```python
from build123d import *

# Parameters (mm, degrees)
F1_DEPTH = 7.62
F2_DEPTH = 1.27
F4_W     = 50.8
F4_H     = 19.067067
F6_W     = 59.465482
F6_H     = 29.439323
F9_DEPTH = 1.27


with BuildPart() as f1:
    # F0 (on Top) → F1 (new body)
    with BuildSketch(Plane.XY):
        Polygon((12.7, 12.7), (-12.7, 12.7), (-12.7, -38.1), (-12.7, -76.2), (12.7, -76.2), (12.7, -38.1), align=None)
        Polygon((12.7, -76.2), (-12.7, -76.2), (0, -127), align=None)
    extrude(amount=F1_DEPTH)

    # F0 (on Top) → F2 (join)
    with BuildSketch(Plane.XY):
        with BuildLine():
            ThreePointArc((139.7, 0), (77.911288, 23.462884), (12.7, 12.7))
            Line((12.7, 12.7), (12.7, -38.1))
            ThreePointArc((12.7, -38.1), (72.718847, -7.994233), (139.7, -12.7))
            Line((139.7, -12.7), (139.7, 0))
        make_face()
        with BuildLine():
            Line((-12.7, -38.1), (-12.7, 12.7))
            ThreePointArc((-12.7, 12.7), (-77.911288, 23.462884), (-139.7, 0))
            Line((-139.7, 0), (-139.7, -12.7))
            ThreePointArc((-139.7, -12.7), (-72.718847, -7.994233), (-12.7, -38.1))
        make_face()
    extrude(amount=F2_DEPTH)

    # F4 (on offset) → F7 section 0
    with BuildSketch(Plane.XZ.offset(76.2)):
        with Locations((0, 17.153533)):
            Rectangle(F4_W, F4_H)
    # F6 (on offset) → F7 section 1
    with BuildSketch(Plane.XZ.offset(127)):
        with Locations((0.102181, 14.719661)):
            Rectangle(F6_W, F6_H)
    loft(mode=Mode.SUBTRACT)

    # F0 (on Top) + F8 (on face) → F9 (join)
    with BuildSketch(Plane.XY):
        Polygon((12.7, -76.2), (-12.7, -76.2), (0, -127), align=None)
    with BuildSketch(Plane.XY):
        Polygon((0, -127), (-12.7, -76.2), (-52.008614, -151.024356), (-52.008614, -167.176113), align=None)
        Polygon((52.008614, -151.024356), (12.7, -76.2), (0, -127), (52.008614, -167.176113), align=None)
    extrude(amount=F9_DEPTH)


solid = f1.part
```
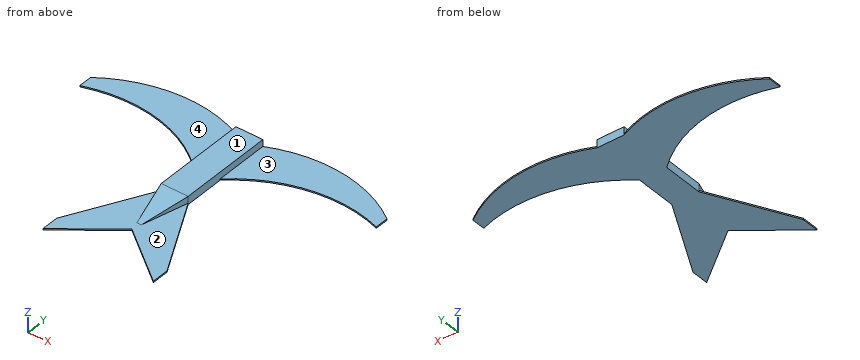
Geometry: final body of the model. Coordinates: model frame, mm. Face numbers are marked on the shaded views. A direction names the side the tool comes from. Coordinates: 2 decimals unless noted, no trailing zeros. Loops run counter-clockwise (first coordinate to the right, second up) from the corner with the lowest first, then second, coordinate; pieces in that order, holes last. Notation, with made-up numbers: (47, 60.25) -> (71, 60.25) arc R18 cw to (71, 86.25) -> close; hole circle Ø8 at (67.5, 48). An arc over 180 degrees is marked (long way). Use a Markdown table: item, result. Add a question column.
(1) Access query for the marked faces 1, 2, 3 and 4. Directions: +Z, -Z, +X, -X, +Y, -Y. A direction counts if a zero-diameter tool reaches every point of the face in a straight line with its end or side. Return the directions, or none.
(2) Section query A-A, the plane x = 16.5. Return loops of the section in (y, z).
(3) Section query D-D, the plane y = -73. Return loops of the section in (x, z), plus the area to 3 significant figures.
(4) Section query C-C, the plane x = 70. Return loops of the section in (y, z).
(5) Section query B-B, the plane y = 4.5. Return loops of the section in (x, z), plus the area to 3 significant figures.
(6) Pin query (flat end, axial travel): pin 1 Ø0.6 at (y, z) = (-162, 0.5) entering from -X; pin 2 Ø4 at (x, z) = (-0.5, 4) entering from +Y; pin 3 Ø1 at (y, z) = (-74, 6) entering from -X; pin 4 Ø3 at (x, z) = (-51, 3.5) entering from -Y. Return the tip coordinate at first contact, or that it passes through.
(7) Line query: line 1 along Z through (x, y) = (-94, 8); line 2 along Y through (x, z) = (-34, 1); line 3 along X through (y, z) = (10.5, 4.5). Output: solid intervals per line, ascending.
Answer:
| question | item | result |
|---|---|---|
| 1 | face 1 | +Z, +X, -X, +Y, -Y |
| 1 | face 2 | +Z, -Y |
| 1 | face 3 | +Z, +X, +Y, -Y |
| 1 | face 4 | +Z, -X, +Y, -Y |
| 2 | outline | (-139.75, 0) -> (-83.43, 0) -> (-83.43, 1.27) -> (-139.75, 1.27) -> close; (-34.82, 0) -> (14.35, 0) -> (14.35, 1.27) -> (-34.82, 1.27) -> close |
| 3 | outline | (-12.7, 0) -> (12.7, 0) -> (12.7, 7.62) -> (-12.7, 7.62) -> close |
| 3 | area | 194 mm^2 |
| 4 | outline | (-8.57, 0) -> (24.01, 0) -> (24.01, 1.27) -> (-8.57, 1.27) -> close |
| 5 | outline | (-133.04, 0) -> (133.04, 0) -> (133.04, 1.27) -> (12.7, 1.27) -> (12.7, 7.62) -> (-12.7, 7.62) -> (-12.7, 1.27) -> (-133.04, 1.27) -> close |
| 5 | area | 499 mm^2 |
| 6 | pin 1 | stops at x = -52.01 |
| 6 | pin 2 | stops at y = 12.7 |
| 6 | pin 3 | stops at x = -12.7 |
| 6 | pin 4 | passes through |
| 7 | line 1 | z = 0 to 1.27 |
| 7 | line 2 | y = -153.26 to -116.74, -22.62 to 20.18 |
| 7 | line 3 | x = -12.7 to 12.7 |
